The listing builds one solid part. Answer for the finished solid, in the listing's coordinates (mm). Give positions to 0.01 mm unless a question says otherwise; leave off trailing zeros. Loops run counter-clockwise (first coordinate to the right, second up) from the corner with the lowest first, then second, coordinate; pieces in that order, holes last.
Item 1: Section B-B, the plane z = 0 is taken. Give the vertices of the cut face in (x, y), and give its area (3 significant figures).
Item 2: Consider line 1 along Z through (x, y) = (0, -28.5); line 2 along Z through (x, y) = (0, -33.75); line 3 along Z through (x, y) = (0, -26). Determine where each line is inside the solid, lowest interval first.
Item 3: The mould has two halves that part along X. Classify faces 1 (the face through (9, -28, -5)), 2 (the face through (-0.443, -23.407, 26.324)), 3 (the face through (-3, -41, 3)): pulls with the +X half, pulls with the -X half, needs draft (parallel to the pull), parting line crosses it, or undercut.
Item 4: Section D-D, the plane z = 31.5 is taken. Give the vertices of the cut face in (x, y), and give its area (3 significant figures).
Item 5: Section A-A, the plane y = -22.5 is taken. Give the number of separate pieces and of enclosed holes in the cut face, and give its area (3 significant figures).
Item 6: Each of these flat-tipped pins is pushed along its axis until it touches: pin 1 Ø10 at (y, z) = (-11, 6) entering from +X; pin 2 Ø5 at (x, z) = (9, -4) entering from -Y; pin 3 Ø6 at (x, y) = (-5.5, -27.5) entering from -Z. Where does it stop, or does it pass through?
Item 7: Section C-C, the plane z = -12.5 is taken. Give the vertices of the cut face in (x, y).
from build123d import *

# Parameters (mm, degrees)
F0_R      = 16.5
F1_DEPTH  = 21
F2_R      = 16.5
F2_R_2    = 13.851235
F3_DEPTH  = 10
F4_R      = 4.8
F4_R_2    = 3.518021
F5_DEPTH  = 20
F7_DEPTH  = 7
F10_R     = 3.4
F10_R_2   = 2.068138
F11_DEPTH = 20


with BuildPart() as f1:
    # F0 (on Front) → F1 (new body)
    with BuildSketch(Plane.XZ):
        Circle(F0_R)
    extrude(amount=F1_DEPTH)

    # F2 (on face) → F3 (join)
    with BuildSketch(Plane.XZ.offset(21)):
        Circle(F2_R)
        Circle(F2_R_2, mode=Mode.SUBTRACT)
    extrude(amount=F3_DEPTH)

    # F4 (on face) → F5 (join)
    with BuildSketch(Plane.XZ.offset(21)):
        Circle(F4_R)
        Circle(F4_R_2, mode=Mode.SUBTRACT)
    extrude(amount=F5_DEPTH)

    # F6 (on face) → F7 (join)
    with BuildSketch(Plane.XZ.offset(21)):
        with BuildLine():
            Line((10.207186, -9.018168), (10.485276, -7.813368))
            ThreePointArc((10.485276, -7.813368), (10.207186, -3.996652), (7.31172, -1.494465))
            Line((7.31172, -1.494465), (5.314166, -0.832571))
            Line((5.314166, -0.832571), (4.465776, -3.392957))
            Line((4.465776, -3.392957), (6.68265, -3.392957))
            ThreePointArc((6.68265, -3.392957), (8.41993, -4.894269), (8.586784, -7.184299))
            Line((8.586784, -7.184299), (7.979127, -9.018168))
            Line((7.979127, -9.018168), (7.979127, -10.589611))
            Line((7.979127, -10.589611), (10.207186, -9.018168))
        make_face()
        with BuildLine():
            ThreePointArc((1.523938, 12.987199), (-1.642391, 10.838008), (-2.361615, 7.079367))
            Line((-2.361615, 7.079367), (-1.936055, 5.018488))
            Line((-1.936055, 5.018488), (0.705499, 5.563954))
            Line((0.705499, 5.563954), (-0.402938, 7.483823))
            ThreePointArc((-0.402938, 7.483823), (0.028596, 9.739007), (1.928393, 11.028522))
            Line((1.928393, 11.028522), (3.820399, 11.419211))
            Line((3.820399, 11.419211), (5.181308, 12.204932))
            Line((5.181308, 12.204932), (2.70637, 13.348766))
            Line((2.70637, 13.348766), (1.523938, 12.987199))
        make_face()
        with BuildLine():
            ThreePointArc((-12.009213, -5.173831), (-8.564795, -6.841356), (-4.950104, -5.584903))
            Line((-4.950104, -5.584903), (-3.378111, -4.185917))
            Line((-3.378111, -4.185917), (-5.171275, -2.170997))
            Line((-5.171275, -2.170997), (-6.279712, -4.090866))
            ThreePointArc((-6.279712, -4.090866), (-8.448526, -4.844738), (-10.515177, -3.844223))
            Line((-10.515177, -3.844223), (-11.799526, -2.401043))
            Line((-11.799526, -2.401043), (-13.160435, -1.615321))
            Line((-13.160435, -1.615321), (-12.913556, -4.330598))
            Line((-12.913556, -4.330598), (-12.009213, -5.173831))
        make_face()
    extrude(amount=F7_DEPTH)

    # F10 (on plane+point) → F11 (join)
    with BuildSketch(Plane.XY.offset(16.464327)):
        with Locations((0, -26.77853)):
            Circle(F10_R)
        with Locations((0, -26.77853)):
            Circle(F10_R_2, mode=Mode.SUBTRACT)
    extrude(amount=F11_DEPTH)


solid = f1.part
Worked answers:
1. outline: (-16.5, -31) - (-13.85, -31) - (-13.85, -21) - (-4.8, -21) - (-4.8, -41) - (-3.52, -41) - (-3.52, -21) - (3.52, -21) - (3.52, -41) - (4.8, -41) - (4.8, -21) - (13.85, -21) - (13.85, -31) - (16.5, -31) - (16.5, 0) - (-16.5, 0) - close
1. area: 797 mm2
2. line 1: z = -16.5 to -13.85, -4.8 to -3.52, 3.52 to 4.8, 13.85 to 16.5
2. line 2: z = -4.8 to -3.52, 3.52 to 4.8
2. line 3: z = -16.5 to -13.85, -4.8 to -3.52, 3.52 to 4.8, 5.42 to 6.79, 9.69 to 12.4, 13.85 to 16.5
3. face 1: undercut
3. face 2: parting line crosses it
3. face 3: needs draft
4. outline: circle Ø6.8 at (0, -26.78); hole circle Ø4.14 at (0, -26.78)
4. area: 22.9 mm2
5. separate pieces: 5
5. enclosed holes: 2
5. area: 354 mm2
6. pin 1: stops at x = 16.47
6. pin 2: stops at y = -28
6. pin 3: stops at z = -16.31
7. outline: (-10.77, -31) - (-5.97, -31) - (-5.97, -21) - (5.97, -21) - (5.97, -31) - (10.77, -31) - (10.77, 0) - (-10.77, 0) - close
